Autodesk Inventor part; units mm, degrees
ref_plane "YZ Plane" through (0, 0, 0) normal (1, 0, 0) x (0, 1, 0)
ref_plane "XZ Plane" through (0, 0, 0) normal (0, 1, 0) x (-1, 0, 0)
ref_plane "XY Plane" through (0, 0, 0) normal (0, 0, 1) x (1, 0, 0)
sketch "Sketch1" plane through (0, 0, 0) normal (0, 0, 1) x (1, 0, 0)
  line L0 (0, 0) -> (19, 0)
  line L1 (19, 0) -> (19, 213)
  line L2 (19, 213) -> (0, 213)
  line L3 (0, 213) -> (0, 0)
  dimension "d0" = 19
  dimension "d1" = 213
extrude "Extrusion1" add sketch "Sketch1" along normal blind 19
sketch "Sketch2" plane through (0, 0, 0) normal (0, -1, 0) x (1, 0, 0)
  line L0 (0, 0) -> (19, 0)
  line L1 (19, 0) -> (19, 19)
  line L2 (0, 19) -> (19, 19)
  line L3 (0, 0) -> (0, 19)
  line L4 (17.5, 17.5) -> (17.5, 1.5)
  line L5 (17.5, 1.5) -> (1.5, 1.5)
  line L6 (1.5, 1.5) -> (1.5, 17.5)
  line L7 (1.5, 17.5) -> (17.5, 17.5)
  dimension "d4" = 1.5
extrude "Extrusion2" cut sketch "Sketch2" against normal through all contours L4 L5 L6 L7
sketch "Sketch3" plane through (0, 0, 19) normal (0, 0, 1) x (1, 0, 0)
  line L0 (9.5, 96.25) -> (9.5, 126.75) construction
  circle A0 centre (9.5, 126.75) radius 3
  circle A1 centre (9.5, 96.25) radius 4.5
  line L1 (19, 0) -> (19, 213)
  line L2 (19, 213) -> (0, 213)
  point P0 (0, 0)
  point P1 (19, 106.5)
  point P2 (9.5, 111.5)
  point P3 (9.5, 213)
  dimension "d7" = 30.5
  dimension "d8" = 6
  dimension "d9" = 9
  dimension "d12" = 5
extrude "Extrusion3" cut sketch "Sketch3" against normal through all
properties part number "C010" material "Aluminum 6061"
CAD build for the part. Positions are in the model's coordinates, mm. A direction names the side the tool comes from. Round coordinates to 2 decimals unless told otherwise and drop trailing zeros. Write each loop counter-clockwise with the first axis right and the second up, starting at its lowest first coordinate (ties: lowest second). Pieces come first, ordered by that corner, then holes.
Item 1: Mould opens along Z. For faces 1 (the cylindrical face through (8.91, 100.71, 0.76)), 2 (the flat face through (9, 108, 0)), 3 (the flat face through (1.5, 105, 9)) say: released by +Z, released by -Z, zero draft, split by the parting line, or undercut.
Filled in:
face 1: zero draft
face 2: released by -Z
face 3: undercut
Item 2: Drill centre lines: L1, parallel to Y at x = 9.5, z = 18.6; L2, parallel to Z at x = 14, y = 120. Where is each one in solid material? Low to high.
Filled in:
L1: y = 0 to 91.75, 100.75 to 123.75, 129.75 to 213
L2: z = 0 to 1.5, 17.5 to 19
Item 3: Band-saw the part on B-B on x = 9.5. Write the cut outline in (y, z).
Filled in:
outline: (0, 0) - (91.75, 0) - (91.75, 1.5) - (0, 1.5) - close; (0, 17.5) - (91.75, 17.5) - (91.75, 19) - (0, 19) - close; (100.75, 0) - (123.75, 0) - (123.75, 1.5) - (100.75, 1.5) - close; (100.75, 17.5) - (123.75, 17.5) - (123.75, 19) - (100.75, 19) - close; (129.75, 0) - (213, 0) - (213, 1.5) - (129.75, 1.5) - close; (129.75, 17.5) - (213, 17.5) - (213, 19) - (129.75, 19) - close
Item 4: Tool access for faces 4 (the flat face through (0, 108, 9)), 5 (the flat face through (10, 105, 1.5)): list every direction of +Z, -Z, +X, -X, +Y, -Y with a clear straight run to the whole face (end or side of a thin tool).
Filled in:
face 4: +Z, -Z, -X, +Y, -Y
face 5: +Y, -Y
Item 5: Band-saw the part on C-C on z = 13. Write the cut outline in (x, y), then the cut area to 3 significant figures.
Filled in:
outline: (0, 0) - (1.5, 0) - (1.5, 213) - (0, 213) - close; (17.5, 0) - (19, 0) - (19, 213) - (17.5, 213) - close
area: 639 mm2
Item 6: Band-saw the part on D-D on y = 61.5. Write the cut outline in (x, z).
Filled in:
outline: (0, 0) - (19, 0) - (19, 19) - (0, 19) - close; hole (1.5, 1.5) - (17.5, 1.5) - (17.5, 17.5) - (1.5, 17.5) - close
Item 7: Band-saw the part on A-A on y = 96.25. Write the cut outline in (x, z), then the cut area to 3 significant figures.
Filled in:
outline: (0, 0) - (5, 0) - (5, 1.5) - (1.5, 1.5) - (1.5, 17.5) - (5, 17.5) - (5, 19) - (0, 19) - close; (14, 0) - (19, 0) - (19, 19) - (14, 19) - (14, 17.5) - (17.5, 17.5) - (17.5, 1.5) - (14, 1.5) - close
area: 78.0 mm2
Item 8: Drop flat-ended pins along their axis: pin 1 Ø2 at (x, y) = (6, 160.5) entering from -Z; pin 2 Ø6 at (x, z) = (9, 12) entering from -Y. Give the stop position or say it passes through.
Filled in:
pin 1: stops at z = 0
pin 2: passes through
